from build123d import *

# Parameters (mm, degrees)
F1_DEPTH = 76.2
F2_R     = 15.3048554067
F3_DEPTH = 63.501
F5_DEPTH = 38.1


# Not quite as in the source:
# - a feature names something its author has since deleted; it is built from what else it names


with BuildPart() as f1:
    # F0 (on Front) → F1 (new body)
    with BuildSketch(Plane.XZ):
        Polygon((-48.8696609855, -52.1779545115), (40.0303390145, -52.1779545115), (40.0303390145, -26.7779545115), (14.6303390145, -26.7779545115), (14.6303390145, 36.7220454885), (40.0303390145, 36.7220454885), (40.0303390145, 62.1220454885), (-48.8696609855, 62.1220454885), (-48.8696609855, 36.7220454885), (-23.4696609855, 36.7220454885), (-23.4696609855, -26.7779545115), (-48.8696609855, -26.7779545115), align=None)
    extrude(amount=F1_DEPTH)

    # F2 (on face) → F3 (cut, through all)
    with BuildSketch(Plane.YZ.offset(14.6303390145)):
        with Locations((-38.1, 4.9720454885)):
            Circle(F2_R)
    extrude(amount=-F3_DEPTH, mode=Mode.SUBTRACT)

    # F4 (on face) → F5 (join)
    with BuildSketch(Plane.XY.offset(62.1220454885)):
        Polygon((-17.6424384117, -63.2961168885), (0, -40.7014116645), (14.5472735167, -40.7014116645), (14.5472735167, -17.7971962839), (-34.9753573537, -17.7971962839), align=None)
    extrude(amount=F5_DEPTH)


solid = f1.part
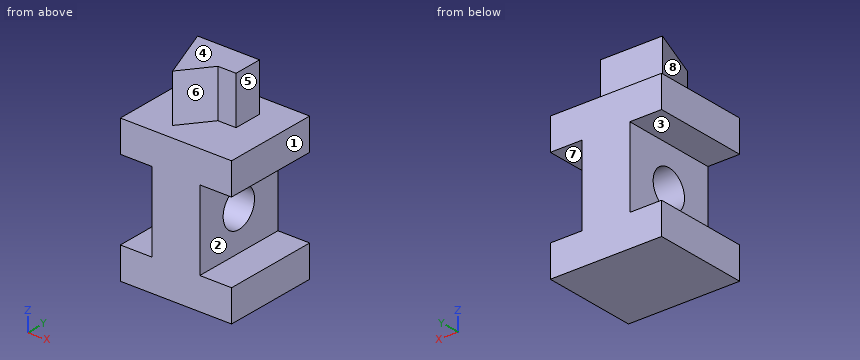
Here's how the part is built. I have some questions about the finished solid (model axes, mm). Face numbers are marked on the shaded views. A direction names the side the tool comes from. Coordinates: 2 decimals unless noted, no trailing zeros. Write each loop counter-clockwise with the first axis right and the second up, starting at its lowest first coordinate (ties: lowest second). Pieces come first, ordered by that corner, then holes.
Item 1: On a 3-axis mill with a long thin cutter (end or side, diameter ignored), from which of +Z, -Z, +X, -X, +Y, -Y can I reach the whole of each face in a straight line? I mean the marked faces 5, 6, 7 and 8. Say none if no direction works.
Item 2: I want a section at A-A on x = -39. Write out the boundary of the cut face in (y, z), and give its area (3 significant figures).
Item 3: I want a section at B-B on y = -37. Write out the boundary of the cut face in (x, z).
Item 4: Will these pins go through, and if not, where does the flat tip stop? pin 1 (3 mm diameter, centred on y = -62, z = 68, fed in from -X); pin 2 (2 mm diameter, centred on x = 26, y = -37.5, fed in from +Z); pin 3 (18.5 mm diameter, centred on y = -25, z = 74, fed in from +X); pin 4 (4 mm diameter, centred on y = -33.5, z = -26, fed in from -X).
Item 5: If I drill on line 1 (Z direction, x = -3, y = -38); line 2 (Z direction, x = -25, y = -37.5); line 3 (Y direction, x = 4, z = 6), over which ranges is the centre line in solid material (lowest first)?
Item 6: I want a section at C-C on z = 11. Write out the boundary of the cut face in (x, y), and give its area (3 significant figures).
Item 7: If we mould it in two halves opening along Z, with no side actions, what happens to the marked faces 1, 2, 3 and 4? For each: +Z half, -Z half, draft (parallel to the pull), parting line (faces both ways), or undercut.
Item 8: I want a section at D-D on x = -14.5. Write out the boundary of the cut face in (y, z), and give its area (3 significant figures).
Findings below:
1. face 5: +Z, +X, +Y, -Y
1. face 6: +Z, +X, -Y
1. face 7: +X, +Y, -Y
1. face 8: +Z, -X, -Y
2. outline: (-76.2, -52.18) - (0, -52.18) - (0, -26.78) - (-76.2, -26.78) - close; (-76.2, 36.72) - (0, 36.72) - (0, 62.12) - (-76.2, 62.12) - close
2. area: 3,870 mm2
3. outline: (-48.87, -52.18) - (40.03, -52.18) - (40.03, -26.78) - (14.63, -26.78) - (14.63, -10.29) - (-23.47, -10.29) - (-23.47, -26.78) - (-48.87, -26.78) - close; (-48.87, 36.72) - (-23.47, 36.72) - (-23.47, 20.24) - (14.63, 20.24) - (14.63, 36.72) - (40.03, 36.72) - (40.03, 62.12) - (14.55, 62.12) - (14.55, 100.22) - (-27.66, 100.22) - (-27.66, 62.12) - (-48.87, 62.12) - close
4. pin 1: stops at x = -18.71
4. pin 2: stops at z = 62.12
4. pin 3: stops at x = 14.55
4. pin 4: stops at x = -48.87
5. line 1: z = -52.18 to -10.33, 20.28 to 100.22
5. line 2: z = -52.18 to -26.78, 36.72 to 100.22
5. line 3: y = -76.2 to -53.37, -22.83 to 0
6. outline: (-23.47, -76.2) - (14.63, -76.2) - (14.63, -52.17) - (-23.47, -52.17) - close; (-23.47, -24.03) - (14.63, -24.03) - (14.63, 0) - (-23.47, 0) - close
6. area: 1,830 mm2
7. face 1: draft
7. face 2: undercut
7. face 3: undercut
7. face 4: +Z half
8. outline: (-76.2, -52.18) - (0, -52.18) - (0, 62.12) - (-17.8, 62.12) - (-17.8, 100.22) - (-59.27, 100.22) - (-59.27, 62.12) - (-76.2, 62.12) - close; hole circle Ø30.61 at (-38.1, 4.97)
8. area: 9,550 mm2
